```python
from build123d import *

# Parameters (mm, degrees)
SKETCH_1_W          = 32
SKETCH_1_H          = 23.5
EXTRUDE_2_DEPTH     = 23.5
SHELL_1_T           = -1.5
FILLET_2_R          = 1.5
SKETCH_3_R          = 2.5
CUT_EXTRUDE_2_DEPTH = 23.5
SKETCH_5_R          = 2.5
CUT_EXTRUDE_3_DEPTH = 23.5


with BuildPart() as part:
    # 草图1 → 凸台-拉伸2 (new body)
    with BuildSketch(Plane.XY):
        with Locations((16, 11.75)):
            Rectangle(SKETCH_1_W, SKETCH_1_H)
    extrude(amount=EXTRUDE_2_DEPTH)

    # 抽壳1
    shell_1_openings = [part.faces().sort_by_distance(p)[0] for p in [
        (16, 11.75, 23.5),
        (32, 11.75, 11.75),
        (16, 0, 11.75),
        (0, 11.75, 11.75),
    ]]
    offset(amount=SHELL_1_T, openings=shell_1_openings, kind=Kind.INTERSECTION)

    # 圆角2
    fillet_2_edges = [part.edges().sort_by_distance(p)[0] for p in [
        (16, 23.5, 0),
    ]]
    fillet(fillet_2_edges, radius=FILLET_2_R)

    # 草图3 → 切除-拉伸2 (cut)
    with BuildSketch(Plane.XY.offset(1.5)):
        with Locations((7.5, 7)):
            Circle(SKETCH_3_R)
        with Locations(Location((24.5, 7, 0), (0, 0, 180))):
            Circle(SKETCH_3_R)
    extrude(amount=-CUT_EXTRUDE_2_DEPTH, mode=Mode.SUBTRACT)

    # 草图5 → 切除-拉伸3 (cut)
    with BuildSketch(Plane.XZ.offset(-22)):
        with Locations(Location((7.5, 16.5, 0), (0, 0, 270))):
            Circle(SKETCH_5_R)
        with Locations(Location((24.5, 16.5, 0), (0, 0, 270))):
            Circle(SKETCH_5_R)
    extrude(amount=-CUT_EXTRUDE_3_DEPTH, mode=Mode.SUBTRACT)


solid = part.part
```
CAD build for the part. Positions are in the model's coordinates, mm. A direction names the side the tool comes from. Round coordinates to 2 decimals unless told otherwise and drop trailing zeros. Order: outer loops, then holes, each group sorted by start corner. A loop starts at its lowest first (then second) coordinate and runs counter-clockwise, first axis right, second up.
Item 1: Saw through at D-D on x = 12. Write the cut outline in (y, z), then the cut area to 3 significant figures.
Item 2: Tool access for faces 4 (the face through (16, 0, 1)), 5 (the face through (16, 11, 1.5)): list every direction of +Z, -Z, +X, -X, +Y, -Y with a clear straight run to the whole face (end or side of a thin tool).
Item 3: Saw through at A-A on z = 16.5. Write the cut outline in (x, y).
Item 4: Saw through at C-C on y = 5.75. Write the cut outline in (x, z), then the cut area to 3 significant figures.
Item 5: Probe line 1 along X through (y, z) = (23.05, 16.5); line 2 along Y through (x, z) = (8.5, 7.5); line 3 along Z through (x, y) = (27, 17.5). List the from-to ranges inside material, lowest first.
Item 6: Saw through at B-B on x = 5.5. Write the cut outline in (y, z).
Item 7: Mould opens along X. For faces 1 (the face through (9.81, 6.04, 0.76)), 2 (the face through (0, 17, 1)), 3 (the face through (16, 22, 12)) say: pulls with the +X half, pulls with the -X half, needs draft (parallel to the pull), parting line crosses it, or undercut.
Item 8: Pin check, flat tips, straight feed: pin 1 (3 mm diameter, centred on x = 9, z = 18.5, fed in from -Y); pin 2 (6.5 mm diameter, centred on x = 18.5, y = 14.5, fed in from +Z); pin 3 (4.5 mm diameter, centred on x = 24.5, y = 7, fed in from -Z). Stop position of each tip, or through.
Reported:
1. outline: (0, 0) - (22, 0) arc R1.5 ccw to (23.5, 1.5) - (23.5, 23.5) - (22, 23.5) - (22, 1.5) - (0, 1.5) - close
1. area: 67.8 mm2
2. face 4: +Z, -Z, +X, -X, -Y
2. face 5: +Z, +X, -X, -Y
3. outline: (0, 22) - (5, 22) - (5, 23.5) - (0, 23.5) - close; (10, 22) - (22, 22) - (22, 23.5) - (10, 23.5) - close; (27, 22) - (32, 22) - (32, 23.5) - (27, 23.5) - close
4. outline: (0, 0) - (5.33, 0) - (5.33, 1.5) - (0, 1.5) - close; (9.67, 0) - (22.33, 0) - (22.33, 1.5) - (9.67, 1.5) - close; (26.67, 0) - (32, 0) - (32, 1.5) - (26.67, 1.5) - close
4. area: 35.0 mm2
5. line 1: x = 0 to 5, 10 to 22, 27 to 32
5. line 2: y = 22 to 23.5
5. line 3: z = 0 to 1.5
6. outline: (0, 0) - (5.5, 0) - (5.5, 1.5) - (0, 1.5) - close; (8.5, 0) - (22, 0) arc R1.5 ccw to (23.5, 1.5) - (23.5, 15) - (22, 15) - (22, 1.5) - (8.5, 1.5) - close; (22, 18) - (23.5, 18) - (23.5, 23.5) - (22, 23.5) - close
7. face 1: undercut
7. face 2: pulls with the -X half
7. face 3: needs draft
8. pin 1: stops at y = 22
8. pin 2: stops at z = 1.5
8. pin 3: passes through
